Autodesk Inventor part; units mm, degrees
ref_plane "YZ Plane" through (0, 0, 0) normal (1, 0, 0) x (0, 1, 0)
ref_plane "XZ Plane" through (0, 0, 0) normal (0, 1, 0) x (-1, 0, 0)
ref_plane "XY Plane" through (0, 0, 0) normal (0, 0, 1) x (1, 0, 0)
sketch "Sketch1" plane through (0, 0, 0) normal (0, 0, 1) x (1, 0, 0)
  line L0 (-197, 62.5) -> (197, 62.5)
  line L1 (197, 62.5) -> (197, -62.5)
  line L2 (197, -62.5) -> (-197, -62.5)
  line L3 (-197, -62.5) -> (-197, 62.5)
  line L4 (-197, 62.5) -> (197, -62.5) construction
  line L5 (197, 62.5) -> (-197, -62.5) construction
  point P0 (0, 0)
  dimension "d0" = 394
  dimension "d1" = 125
extrude "Extrusion1" add sketch "Sketch1" against normal blind 3
sketch "Sketch2" plane through (0, 0, 0) normal (0, 0, 1) x (1, 0, 0)
  circle A0 centre (-157, -22.5) radius 10
  circle A1 centre (-117, -22.5) radius 10
  line L0 (-197, -62.5) -> (197, -62.5)
  line L1 (-197, 62.5) -> (-197, -62.5)
  line L2 (37, 45.5) -> (107, 45.5)
  line L3 (112, 40.5) -> (112, -12.5)
  line L4 (107, -17.5) -> (37, -17.5)
  line L5 (32, -12.5) -> (32, 40.5)
  line L6 (197, 62.5) -> (-197, 62.5)
  line L7 (197, -62.5) -> (197, 62.5)
  arc A2 (37, 45.5) -> (32, 40.5) centre (37, 40.5) ccw
  arc A3 (112, 40.5) -> (107, 45.5) centre (107, 40.5) ccw
  arc A4 (107, -17.5) -> (112, -12.5) centre (107, -12.5) ccw
  arc A5 (32, -12.5) -> (37, -17.5) centre (37, -12.5) ccw
  point P0 (0, 0)
  point P1 (32, 45.5)
  point P2 (112, -17.5)
  point P3 (112, 45.5)
  point P4 (32, -17.5)
  dimension "d4" = 20
  dimension "USB" = 20
  dimension "d6" = 40
  dimension "d7" = 40
  dimension "d8" = 40
  dimension "d9" = 40
  dimension "d10" = 63
  dimension "d11" = 17
  dimension "d12" = 80
  dimension "d13" = 85
  dimension "d16" = 5
extrude "Extrusion2" cut sketch "Sketch2" against normal blind 3 contours A0 | A1 | L2 A3 L3 A4 L4 A5 L5 A2
equation "\"d4\" = USB"
properties part number "BackPanel"
Read the model definition and answer for the solid it produces. Units are mm, in the model's axes. Round coordinates to 2 decimals unless told otherwise and drop trailing zeros. Order: outer loops, then holes, each group sorted by start corner. A loop starts at its lowest first (then second) coordinate and runs counter-clockwise, first axis right, second up. Notation, with made-up numbers: (-35, -13) - (15, -13) arc R17 cw to (15, -2) - close; hole circle Ø10 at (36.25, 19.5). An arc over 180 degrees is marked (long way). Use one line per item in the form item = value. Start each with the question number.
(1) The part is cut by section A-A (x = 62.5). Give the vertices of the cut face in (y, z), then the cut area to 3 significant figures.
(2) The part is cut by section B-B (y = -9). Give the vertices of the cut face in (x, z), then the cut area to 3 significant figures.
(3) A flat-ended cylindrical pin translates along its axis: pin 1 Ø3 at (x, y) = (118.5, 30) entering from +Z. Find the tip coordinate at first contact, or state that the pin passes through.
(4) Find the intervals of material crossed by line 1 along X through (y, z) = (2, -2.1); line 2 along Y through (x, z) = (40, -2.55); line 3 along Y through (x, z) = (-157, -1.95), in increasing order. Write a range as from..to.
(5) The part is cut by section C-C (z = -2.4). Give the vertices of the cut face in (x, y), then the cut area to 3 significant figures.
(6) Determine the mould class of faces 1 (the face through (-3, 1, -3)), 2 (the face through (-124.37, -15.74, -1.48)) for opening direction X: +X half, -X half, draft (parallel to the pull), parting line (faces both ways), or undercut.
Checked values:
q1.outline = (-62.5, -3) - (-17.5, -3) - (-17.5, 0) - (-62.5, 0) - close; (45.5, -3) - (62.5, -3) - (62.5, 0) - (45.5, 0) - close
q1.area = 186 mm^2
q2.outline = (-197, -3) - (32, -3) - (32, 0) - (-197, 0) - close; (112, -3) - (197, -3) - (197, 0) - (112, 0) - close
q2.area = 942 mm^2
q3.pin_1 = 0
q4.line_1 = -197..32, 112..197
q4.line_2 = -62.5..-17.5, 45.5..62.5
q4.line_3 = -62.5..-32.5, -12.5..62.5
q5.outline = (-197, -62.5) - (197, -62.5) - (197, 62.5) - (-197, 62.5) - close; hole circle Ø20 at (-157, -22.5); hole circle Ø20 at (-117, -22.5); hole (32, -12.5) arc R5 ccw to (37, -17.5) - (107, -17.5) arc R5 ccw to (112, -12.5) - (112, 40.5) arc R5 ccw to (107, 45.5) - (37, 45.5) arc R5 ccw to (32, 40.5) - close
q5.area = 43,600 mm^2
q6.face_1 = draft
q6.face_2 = undercut
